Geometry: final body of the model. Coordinates: model frame, mm. A direction names the side the tool comes from. Round coordinates to 2 decimals unless told otherwise and drop trailing zeros. Write each loop counter-clockwise with the first axis right and the second up, starting at its lowest first coordinate (ties: lowest second). Pieces come first, ordered by that corner, then holes. Notation, with made-up numbers: M -16.5,-1.75 L 39.5,-1.75 A34 cw 39.5,31.25 Z; hole C 47.25,-18.5 d5. An arc over 180 degrees is marked long. Answer as CSV lines item,"result". Start each with the question number.
Q1. Section query C-C on x = -0.25. Output: boundary loops of the cut face in (y, z), and give its area (3 significant figures).
Q2. First-contact query: pin 1 (1.1 mm diameter, centred on x = 1, z = 194, fed in from +Y); pin 2 (0.5 mm diameter, centred on x = -3, z = 189, fed in from +Y); pin 3 (1.7 mm diameter, centred on x = 0, z = 174.5, fed in from -Y). Flat tips, straight axial feed; report the tip coordinate or a pass-through.
Q3. Section query B-B on z = 188.5. Output: boundary loops of the cut face in (x, y) (3 decimals).
Q4. Reachability of faces 5 (the flat face through (-0.34, -1.11, 226.25)), 6 (the flat face through (0, -1.283, 182)), 7 (the flat face through (4.025, -1, 182)) from +Z, -Z, +X, -X, +Y, -Y: full face, straight path, thin tool, end or side. Return the list, or none.
Q5. Ray query, probe 1 along X at (y, z) = (-0.5, 142.5); probe 2 along Y at (x, z) = (1.5, 140.5); probe 3 along Y at (x, z) = (2.5, 162.5). Return the intervals inside material, ascending.
Q6. Mould query, pull axis X, two halves, no side actions, for faces 1 (the flat face through (0, -0.958, 182)), 2 (the flat face through (-4.35, -1, 182)), 3 (the flat face through (3, -2.057, 182)), 4 (the flat face through (-4.025, -1, 182)). Classes: pulls with the +X half, pulls with the -X half, needs draft (parallel to the pull), parting line crosses it, or undercut.
Q7. Section query A-A on y = -0.45. Output: boundary loops of the cut face in (x, z), and give its area (3 significant figures).
```python
from build123d import *

# Parameters (mm, degrees)
BOSS_EXTRUDE1_DEPTH = 362
SCALE1_SCALE        = 0.25


with BuildPart() as part:
    # Sketch1 → Boss-Extrude1 (new body)
    with BuildSketch(Plane.XY.offset(362)):
        Polygon((-9.180453293, -3.095455134), (-16.1, -3.095455134), (-16.1, 5.304544866), (-17.4, 5.304544866), (-17.4, -4.395455134), (-8.4, -4.395455134), (-6.749887033, -1.3), (6.750112967, -1.3), (8.4, -4.395455134), (17.4, -4.395455134), (17.4, 5.304544866), (16.1, 5.304544866), (16.1, -3.095455134), (9.18022736, -3.095455134), (7.530340327, 0), (-7.530340327, 0), align=None)
    extrude(amount=-BOSS_EXTRUDE1_DEPTH)


with BuildPart() as part_1:
    # Scale1: scaled about (-7.7465e-05, -1.277039924, 181)
    add(part.part.scale(SCALE1_SCALE).moved(Location((-5.8099e-05, -0.957779943, 135.75))))


solid = part_1.part
```
Entries:
1,outline,"M -1.28,135.75 L -0.96,135.75 L -0.96,226.25 L -1.28,226.25 Z"
1,area,"29.4 mm^2"
2,pin 1,"stops at y = -0.96"
2,pin 2,"stops at y = -1.73"
2,pin 3,"stops at y = -1.28"
3,outline,"M -4.35,-2.057 L -2.1,-2.057 L -1.688,-1.283 L 1.687,-1.283 L 2.1,-2.057 L 4.35,-2.057 L 4.35,0.368 L 4.025,0.368 L 4.025,-1.732 L 2.295,-1.732 L 1.883,-0.958 L -1.883,-0.958 L -2.295,-1.732 L -4.025,-1.732 L -4.025,0.368 L -4.35,0.368 Z"
4,face 5,"+Z, +X, -X, +Y, -Y"
4,face 6,"+Z, -Z, -Y"
4,face 7,"+Z, -Z, +Y"
5,probe 1,"x = -4.35 to -4.03, 4.02 to 4.35"
5,probe 2,"y = -1.28 to -0.96"
5,probe 3,"y = -2.06 to -1.73"
6,face 1,"undercut"
6,face 2,"pulls with the -X half"
6,face 3,"needs draft"
6,face 4,"undercut"
7,outline,"M -4.35,135.75 L -4.03,135.75 L -4.03,226.25 L -4.35,226.25 Z; M 4.02,135.75 L 4.35,135.75 L 4.35,226.25 L 4.02,226.25 Z"
7,area,"58.8 mm^2"
